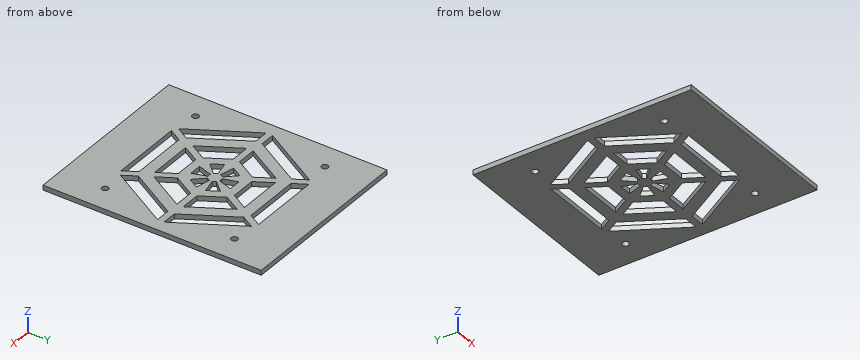
from build123d import *

# Parameters (mm, degrees)
SKETCH1_W           = 111.25
SKETCH1_H           = 135
BOSS_EXTRUDE1_DEPTH = 3
SKETCH2_R           = 2
CUT_EXTRUDE2_DEPTH  = 10


with BuildPart() as part:
    # Sketch1 → Boss-Extrude1 (new body)
    with BuildSketch(Plane.XY):
        with Locations((-55.625, 8.729765013)):
            Rectangle(SKETCH1_W, SKETCH1_H)
    extrude(amount=BOSS_EXTRUDE1_DEPTH)

    # Sketch2 → Cut-Extrude2 (cut)
    with BuildSketch(Plane.XY.offset(3)):
        Polygon((-81.342935317, 49.274535649), (-103.59676902, 10.729765013), (-94.470299462, 10.729765013), (-76.779700538, 41.370781164), align=None)
        Polygon((-37.934401077, 43.370781164), (-73.315598923, 43.370781164), (-77.878833702, 51.274535649), (-33.371166298, 51.274535649), align=None)
        Polygon((-16.779700538, 10.729765013), (-34.470299462, 41.370781164), (-29.907064683, 49.274535649), (-7.65323098, 10.729765013), align=None)
        Polygon((-29.907064683, -31.815005622), (-7.65323098, 6.729765013), (-16.779700538, 6.729765013), (-34.470299462, -23.911251138), align=None)
        Polygon((-77.878833702, -33.815005622), (-73.315598923, -25.911251138), (-37.934401077, -25.911251138), (-33.371166298, -33.815005622), align=None)
        Polygon((-103.59676902, 6.729765013), (-81.342935317, -31.815005622), (-76.779700538, -23.911251138), (-94.470299462, 6.729765013), align=None)
        Polygon((-66.779700538, 24.050273089), (-74.470299462, 10.729765013), (-86.531050208, 10.729765013), (-72.810075912, 34.495189624), align=None)
        Polygon((-74.470299462, 6.729765013), (-66.779700538, -6.590743063), (-72.810075912, -17.035659598), (-86.531050208, 6.729765013), align=None)
        Polygon((-47.934401077, -8.590743063), (-41.904025704, -19.035659598), (-69.345974296, -19.035659598), (-63.315598923, -8.590743063), align=None)
        Polygon((-38.439924088, -17.035659598), (-44.470299462, -6.590743063), (-36.779700538, 6.729765013), (-24.718949792, 6.729765013), align=None)
        Polygon((-36.779700538, 10.729765013), (-44.470299462, 24.050273089), (-38.439924088, 34.495189624), (-24.718949792, 10.729765013), align=None)
        Polygon((-47.934401077, 26.050273089), (-63.315598923, 26.050273089), (-69.345974296, 36.495189624), (-41.904025704, 36.495189624), align=None)
        Polygon((-54.482668179, 12.406598332), (-51.84377359, 20.900431181), (-59.40622641, 20.900431181), (-56.767331821, 12.406598332), align=None)
        Polygon((-58.238065149, 11.557470049), (-64.274492877, 18.089736226), (-68.055719287, 11.540459968), (-59.38039697, 9.578893296), align=None)
        Polygon((-59.38039697, 7.88063673), (-68.055719287, 5.919070058), (-64.274492877, -0.630206199), (-58.238065149, 5.902059977), align=None)
        Polygon((-56.767331821, 5.052931694), (-59.40622641, -3.440901155), (-51.84377359, -3.440901155), (-54.482668179, 5.052931694), align=None)
        Polygon((-53.011934851, 5.902059977), (-46.975507123, -0.630206199), (-43.194280713, 5.919070058), (-51.86960303, 7.88063673), align=None)
        Polygon((-51.86960303, 9.578893296), (-43.194280713, 11.540459968), (-46.975507123, 18.089736226), (-53.011934851, 11.557470049), align=None)
        with Locations((-15.625, -31.270234987)):
            Circle(SKETCH2_R)
        with Locations((-95.625, -31.270234987)):
            Circle(SKETCH2_R)
        with Locations((-95.625, 48.729765013)):
            Circle(SKETCH2_R)
        with Locations((-15.625, 48.729765013)):
            Circle(SKETCH2_R)
    extrude(amount=-CUT_EXTRUDE2_DEPTH, mode=Mode.SUBTRACT)


solid = part.part
The listing builds one solid part. Answer for the finished solid, in the listing's coordinates (mm). Give positions to 0.01 mm unless a question says otherwise; leave off trailing zeros. One line per question, with ' | ' between items. Start each with the question number.
1. Find the intervals of material crossed by probe 1 along X at (y, z) = (41, 2.4); probe 2 along Y at (x, z) = (-15.5, 1.75); probe 3 along Y at (x, z) = (-15, 0.7), in increasing order.
2. Given pin 1 Ø5 at (x, y) = (-95.62, -31.27) entering from +Z, flat-ended and moving along its own axis, determine where the tip first touches the part or whether it passes through.
3. Section A-A (z = 1.5) is taken. State how many separate pieces and enclosed holes the cut face has, plus the area to 3 significant figures.
Response values:
1) probe 1: -111.25 to -86.12, -76.99 to -34.26, -25.13 to 0 | probe 2: -58.77 to -33.27, -29.27 to -6.86, 6.73 to 10.73, 24.32 to 46.73, 50.73 to 76.23 | probe 3: -58.77 to -33.17, -29.37 to -6, 6.73 to 10.73, 23.45 to 46.83, 50.63 to 76.23
2) pin 1: z = 3
3) separate pieces: 1 | enclosed holes: 22 | area: 11,500 mm2
